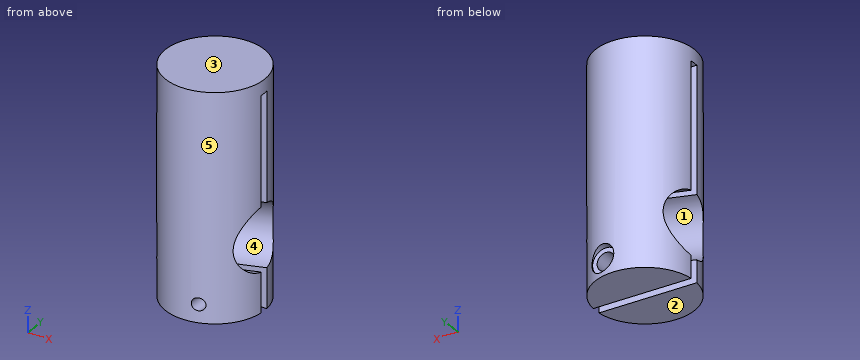
```python
from build123d import *

# Parameters (mm, degrees)
CYLINDER004_R               = 3
CYLINDER004_DEPTH           = 28
CYLINDER003_R               = 2
CYLINDER003_DEPTH           = 28
CYLINDER002_R               = 1.4
CYLINDER002_DEPTH           = 28
BOX_W                       = 100
BOX_H                       = 2
BOX_DEPTH                   = 100
CYLINDER001_R               = 7
CYLINDER001_DEPTH           = 100
CYLINDER001_PLACEMENT_ANGLE = 80
CYLINDER_R                  = 11
CYLINDER_DEPTH              = 50


with BuildPart() as cylinder004:
    # Cylinder004 → Cylinder004 (new body)
    with BuildSketch(Plane(origin=(3, 37, 4), x_dir=(1, 0, 0), z_dir=(0, -1, 0))):
        Circle(CYLINDER004_R)
    extrude(amount=CYLINDER004_DEPTH)


with BuildPart() as cylinder003:
    # Cylinder003 → Cylinder003 (new body)
    with BuildSketch(Plane(origin=(3, 28, 4), x_dir=(1, 0, 0), z_dir=(0, -1, 0))):
        Circle(CYLINDER003_R)
    extrude(amount=CYLINDER003_DEPTH)


with BuildPart() as cylinder002:
    # Cylinder002 → Cylinder002 (new body)
    with BuildSketch(Plane(origin=(3, 13, 4), x_dir=(1, 0, 0), z_dir=(0, -1, 0))):
        Circle(CYLINDER002_R)
    extrude(amount=CYLINDER002_DEPTH)


with BuildPart() as cube:
    # Box → Box (new body)
    with BuildSketch(Plane(origin=(-17, -1, -53), x_dir=(1, 0, 0), z_dir=(0, 0, 1))):
        with Locations((50, 1)):
            Rectangle(BOX_W, BOX_H)
    extrude(amount=BOX_DEPTH)


with BuildPart() as cylinder001:
    # Cylinder001 → Cylinder001 (new body)
    with BuildSketch(Plane.XY):
        Circle(CYLINDER001_R)
    extrude(amount=CYLINDER001_DEPTH)


with BuildPart() as cylinder001_1:
    # Cylinder001 placement: moved
    add(cylinder001.part.moved(Location((-28, 0, 9))).rotate(Axis((-28, 0, 9), (0, 1, 0)), CYLINDER001_PLACEMENT_ANGLE))


with BuildPart() as cut004:
    # Cylinder → Cylinder (new body)
    with BuildSketch(Plane.XY):
        Circle(CYLINDER_R)
    extrude(amount=CYLINDER_DEPTH)

    # Cut: cut Cylinder001
    add(cylinder001_1.part, mode=Mode.SUBTRACT)

    # Cut001: cut Cube
    add(cube.part, mode=Mode.SUBTRACT)

    # Cut002: cut Cylinder002
    add(cylinder002.part, mode=Mode.SUBTRACT)

    # Cut003: cut Cylinder003
    add(cylinder003.part, mode=Mode.SUBTRACT)

    # Cut004: cut Cylinder004
    add(cylinder004.part, mode=Mode.SUBTRACT)


solid = cut004.part
```
Check sheet for the modelled part. Datum: model origin and axes. Units: mm. Face numbers are marked on the shaded views. A direction names the side the tool comes from. Round coordinates to 2 decimals unless told otherwise and drop trailing zeros. Loops run counter-clockwise (first coordinate to the right, second up) from the corner with the lowest first, then second, coordinate; pieces in that order, holes last. Notation, with made-up numbers: (4, 1) -> (8, 1) arc R12 ccw to (8, 9) -> close; hole circle Ø1 at (18, 34.5). An arc over 180 degrees is marked (long way). Write item = value, one per line. Start each with the question number.
1) Sectioned sample at A-A, the plane y = 1.5. Record the cut outline in (x, z), plus the area to 3 significant figures.
2) Thickness scan on probe 1 along Y at (x, z) = (0.5, 29); probe 2 along Z at (x, y) = (3, 10.45); probe 3 along Y at (x, z) = (2.25, 38). Record the ranges inside material, lowest first.
3) Sectioned sample at B-B, the plane z = 32.5. Record the cut outline in (x, y), plus the area to 3 significant figures.
4) Gauge pin test, flat ends, axial feed: pin 1 Ø2.5 at (x, z) = (-5, 6) entering from +Y; pin 2 Ø5 at (x, z) = (3.5, 4.5) entering from +Y; pin 3 Ø2 at (x, y) = (-1, 0.5) entering from -Z; pin 4 Ø4 at (x, z) = (-5.5, 14) entering from +Y. Record the tip position at first contact, or that the pin passes through.
5) Sectioned sample at D-D, the plane y = 6. Record the cut outline in (x, z), plus the area to 3 significant figures.
6) Release check for a two-part mould opening along Z. For the marked faces 1, 2 and 3 record: released by +Z, released by -Z, zero draft, split by the parting line, or undercut.
7) Sectioned sample at C-C, the plane z = 4. Record the cut outline in (x, y).
8) Set-up check for the marked faces 4 and 5: record each of +Z, -Z, +X, -X, +Y, -Y from which the full face is reachable in a straight line by a thin tool's end or side.
Results are:
q1.outline = (-10.9, 0) -> (10.9, 0) -> (10.9, 8.92) -> (-10.9, 5.07) -> close; (-10.9, 18.96) -> (10.9, 22.8) -> (10.9, 50) -> (-10.9, 50) -> close; hole circle Ø4 at (3, 4)
q1.area = 775 mm^2
q2.probe_1 = -10.99 to -1, 1 to 10.99
q2.probe_2 = 0 to 1, 7 to 50
q2.probe_3 = -10.77 to -1, 1 to 10.77
q3.outline = (-10.95, -1) arc R11 ccw to (10.95, -1) -> close; (-10.95, 1) -> (10.95, 1) arc R11 ccw to start
q3.area = 336 mm^2
q4.pin_1 = 10.34
q4.pin_2 = 10.51
q4.pin_3 = 0
q4.pin_4 = 10.43
q5.outline = (-9.22, 0) -> (9.22, 0) -> (9.22, 11.9) -> (-9.22, 8.65) -> close; (-9.22, 15.97) -> (9.22, 19.22) -> (9.22, 50) -> (-9.22, 50) -> close; hole circle Ø4 at (3, 4)
q5.area = 774 mm^2
q6.face_1 = undercut
q6.face_2 = released by -Z
q6.face_3 = released by +Z
q7.outline = (-10.95, -1) arc R11 ccw to (1.6, -10.88) -> (1.6, -1) -> close; (-10.95, 1) -> (1, 1) -> (1, 9) -> (0, 9) -> (0, 11) arc R11 ccw to start; (4.4, -10.08) arc R11 ccw to (10.95, -1) -> (4.4, -1) -> close; (5, 1) -> (10.95, 1) arc R11 ccw to (6, 9.22) -> (6, 9) -> (5, 9) -> close
q8.face_4 = none
q8.face_5 = +Z, -Z
